Geometry: final body of the model. Coordinates: model frame, mm. Face numbers are marked on the shaded views. A direction names the side the tool comes from. Give positions to 0.01 mm unless a question says otherwise; leave off trailing zeros. Loops run counter-clockwise (first coordinate to the right, second up) from the corner with the lowest first, then second, coordinate; pieces in that order, holes last. Notation, with made-up numbers: (-22, -2.75) - (26, -2.75) arc R21 cw to (26, 10.25) - close; hole circle Ø10 at (59, -0.75). An arc over 180 degrees is marked (long way). Answer in a Markdown table with one row per item.
from build123d import *

# Parameters (mm, degrees)
SKETCH1_W           = 19.05
SKETCH1_H           = 19.05
BOSS_EXTRUDE1_DEPTH = 27.94
SKETCH2_W           = 25.4
SKETCH2_H           = 25.4
BOSS_EXTRUDE2_DEPTH = 3.175
SKETCH3_R           = 5.461
CUT_EXTRUDE1_DEPTH  = 41.291237881
SKETCH4_R           = 9.906
BOSS_EXTRUDE3_DEPTH = 3.175
FILLET1_R           = 1.27
CHAMFER1_SIZE       = 2.54


with BuildPart() as part:
    # Sketch1 → Boss-Extrude1 (new body)
    with BuildSketch(Plane(origin=(0, 0, 0), x_dir=(1, 0, 0), z_dir=(0, 1, 0))):
        Rectangle(SKETCH1_W, SKETCH1_H)
    extrude(amount=BOSS_EXTRUDE1_DEPTH)

    # Sketch2 → Boss-Extrude2 (add)
    with BuildSketch(Plane(origin=(0, 27.94, 0), x_dir=(1, 0, 0), z_dir=(0, 1, 0))):
        Rectangle(SKETCH2_W, SKETCH2_H)
    extrude(amount=BOSS_EXTRUDE2_DEPTH)

    # Sketch3 → Cut-Extrude1 (cut, through all)
    with BuildSketch(Plane(origin=(9.525, 0, 0), x_dir=(0, 0, -1), z_dir=(1, 0, 0))):
        with Locations((0, 15.24)):
            Circle(SKETCH3_R)
    extrude(amount=-CUT_EXTRUDE1_DEPTH, mode=Mode.SUBTRACT)

    # Sketch4 → Boss-Extrude3 (add, symmetric)
    with BuildSketch(Plane(origin=(0, 0, 0), x_dir=(0, 0, -1), z_dir=(1, 0, 0))):
        with Locations((0, 31.115)):
            Circle(SKETCH4_R)
    extrude(amount=BOSS_EXTRUDE3_DEPTH, both=True)

    # Fillet1
    fillet1_edges = [part.edges().sort_by_distance(p)[0] for p in [
        (0, 31.115, 12.7),
        (12.7, 31.115, 0),
        (0, 31.115, -12.7),
        (-12.7, 31.115, 0),
        (-3.175, 31.115, 0),
        (0, 31.115, 9.906),
        (0, 31.115, -9.906),
        (3.175, 31.115, 0),
        (-3.175, 41.021, 0),
        (3.175, 41.021, 0),
    ]]
    fillet(fillet1_edges, radius=FILLET1_R)

    # Chamfer1
    chamfer1_edges = [part.edges().sort_by_distance(p)[0] for p in [
        (0, 0, 9.525),
        (-9.525, 0, 0),
        (0, 0, -9.525),
        (9.525, 0, 0),
    ]]
    chamfer(chamfer1_edges, length=CHAMFER1_SIZE)


solid = part.part
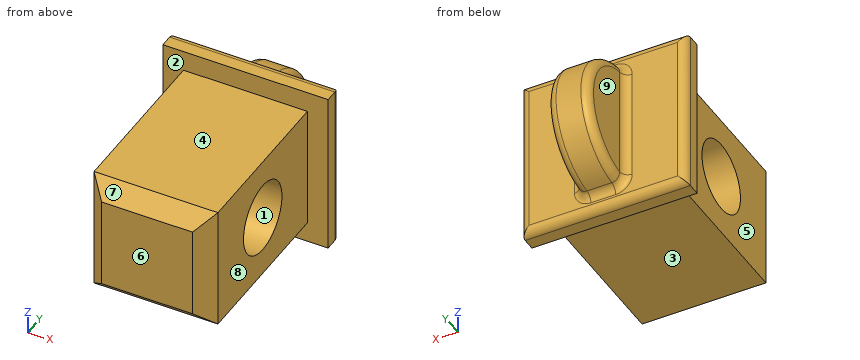
Q1. Draft query along Z for the marked faces 1, 2, 3 and 4. Return one class per face: pulls with the +Z half, pulls with the -Z half, needs draft (parallel to the pull), parting line crosses it, or undercut.
Check values:
| item | result |
|---|---|
| face 1 | undercut |
| face 2 | needs draft |
| face 3 | pulls with the -Z half |
| face 4 | pulls with the +Z half |
Q2. Reachability of the marked faces 5, 6, 7, 8 and 9 from +Z, -Z, +X, -X, +Y, -Y: full face, straight path, thin tool, end or side. Return the list, or none.
Check values:
| item | result |
|---|---|
| face 5 | +Z, -Z, -X, -Y |
| face 6 | +Z, -Z, +X, -X, -Y |
| face 7 | +Z, +X, -X, -Y |
| face 8 | +Z, -Z, +X, -Y |
| face 9 | +Z, -Z, -X, +Y |
Q3. Material intervals for line 1 along Y through (x, z) = (5, 0) (3 decimals); line 2 along Z through (x, y) = (-7, 15) (3 decimals); line 3 along Y through (x, z) = (-11.5, -11.5), sorted ascending.
Check values:
| item | result |
|---|---|
| line 1 | 0 to 9.779, 20.701 to 31.115 |
| line 2 | -9.525 to -5.456, 5.456 to 9.525 |
| line 3 | 27.94 to 31.11 |
Q4. Cut plane C-C (y = 7.5). Output: boundary loops of the cut face in (x, z) (3 decimals).
Check values:
| item | result |
|---|---|
| outline | (-9.525, -9.525) - (9.525, -9.525) - (9.525, 9.525) - (-9.525, 9.525) - close |
Q5. Cut plane B-B (z = 0). Output: boundary loops of the cut face in (x, y) (3 decimals).
Check values:
| item | result |
|---|---|
| outline | (-12.7, 27.94) - (-9.525, 27.94) - (-9.525, 20.701) - (9.525, 20.701) - (9.525, 27.94) - (12.7, 27.94) - (12.7, 29.845) arc R1.27 ccw to (11.43, 31.115) - (4.445, 31.115) arc R1.27 cw to (3.175, 32.385) - (3.175, 39.751) arc R1.27 ccw to (1.905, 41.021) - (-1.905, 41.021) arc R1.27 ccw to (-3.175, 39.751) - (-3.175, 32.385) arc R1.27 cw to (-4.445, 31.115) - (-11.43, 31.115) arc R1.27 ccw to (-12.7, 29.845) - close; (-9.525, 2.54) - (-6.985, 0) - (6.985, 0) - (9.525, 2.54) - (9.525, 9.779) - (-9.525, 9.779) - close |
Q6. First-contact query: pin 1 (3.5 mm diameter, centred on y = 35, z = -3, fed in from -X) (3 decimals); pin 2 (14 mm diameter, centred on y = 15.24, z = 0, fed in from +X) (3 decimals); pin 3 (6 mm diameter, centred on x = -4.5, z = 7.5, fed in from -Y); pin 4 (2 mm diameter, centred on y = 4, z = 0.5, fed in from -X) (3 decimals). Flat tips, straight axial feed; report the tip coordinate or a pass-through.
Check values:
| item | result |
|---|---|
| pin 1 | x = -3.175 |
| pin 2 | x = 9.525 |
| pin 3 | y = 0 |
| pin 4 | x = -9.525 |
Q7. Cut plane A-A (y = 15.24). Output: boundary loops of the cut face in (x, z) (3 decimals), and give its area (3 significant figures).
Check values:
| item | result |
|---|---|
| outline | (-9.525, -9.525) - (9.525, -9.525) - (9.525, -5.461) - (-9.525, -5.461) - close; (-9.525, 5.461) - (9.525, 5.461) - (9.525, 9.525) - (-9.525, 9.525) - close |
| area | 155 mm² |
